```python
from build123d import *

# Parameters (mm, degrees)
F0_R     = 6.5
F1_DEPTH = 3


with BuildPart() as f1:
    # F0 (on Top) → F1 (new body)
    with BuildSketch(Plane.XY):
        with BuildLine():
            Line((0, 64.92969), (0, 105))
            ThreePointArc((0, 105), (-102.329905, 23.528505), (-45.860375, -94.455418))
            Line((-45.860375, -94.455418), (-26.848407, -75.44345))
            Line((-26.848407, -75.44345), (0, -75.44345))
            Line((0, -75.44345), (0, -45.946423))
            Line((0, -45.946423), (-4.373633, -45.946423))
            Line((-4.373633, -45.946423), (-8.012874, -43.948987))
            Line((-8.012874, -43.948987), (-8.012874, -40.483214))
            Line((-8.012874, -40.483214), (-7.424269, -39.663567))
            Line((-7.424269, -39.663567), (-23.331161, -42.38735))
            Line((-23.331161, -42.38735), (-33.173094, -41.479423))
            Line((-33.173094, -41.479423), (-35.896877, -38.101933))
            Line((-35.896877, -38.101933), (-34.589463, -35.37815))
            Line((-34.589463, -35.37815), (-37.494832, -32.944905))
            Line((-37.494832, -32.944905), (-40.373584, -28.384436))
            Line((-40.373584, -28.384436), (-39.757261, -25.662348))
            Line((-39.757261, -25.662348), (-30.409717, -16.543746))
            Line((-30.409717, -16.543746), (-28.680348, -16.543746))
            Line((-28.680348, -16.543746), (-27.497232, -17.393365))
            Line((-27.497232, -17.393365), (-27.497232, -5.479778))
            Line((-27.497232, -5.479778), (-32.618854, -5.479778))
            Line((-32.618854, -5.479778), (-32.618854, 5.955574))
            Line((-32.618854, 5.955574), (-27.497232, 5.955574))
            Line((-27.497232, 5.955574), (-27.497232, 30.408693))
            Line((-27.497232, 30.408693), (-30.054469, 38.053981))
            Line((-30.054469, 38.053981), (-16.39924, 35.148612))
            Line((-16.39924, 35.148612), (-21.810488, 39.03454))
            Line((-21.810488, 39.03454), (-21.810488, 43.537862))
            Line((-21.810488, 43.537862), (-24.057509, 47.911971))
            Line((-24.057509, 47.911971), (-25.507802, 47.911971))
            Line((-25.507802, 47.911971), (-27.497232, 52.08861))
            Line((-27.497232, 52.08861), (-26.29794, 52.65986))
            Line((-26.29794, 52.65986), (-27.144464, 54.437064))
            Line((-27.144464, 54.437064), (-23.446245, 56.198612))
            Line((-23.446245, 56.198612), (-21.478997, 54.78589))
            Line((-21.478997, 54.78589), (-20.486095, 54.78589))
            Line((-20.486095, 54.78589), (-20.000346, 54.437064))
            Line((-20.000346, 54.437064), (-14.9056, 55.777782))
            Line((-14.9056, 55.777782), (-14.033989, 61.988003))
            Line((-14.033989, 61.988003), (-10.583865, 57.266784))
            Line((-10.583865, 57.266784), (-4.373633, 58.90105))
            Line((-4.373633, 58.90105), (-4.373633, 60.244786))
            Line((-4.373633, 60.244786), (-2.230932, 60.244786))
            Line((-2.230932, 60.244786), (-2.230932, 64.92969))
            Line((-2.230932, 64.92969), (0, 64.92969))
        make_face()
        with Locations((-92.039506, -23.116552)):
            Circle(F0_R, mode=Mode.SUBTRACT)
        with Locations((-30.448022, 90.125876)):
            Circle(F0_R, mode=Mode.SUBTRACT)
        with BuildLine():
            ThreePointArc((45.134783, 94.804279), (23.136018, 102.419357), (0, 105))
            Line((0, 105), (0, 64.92969))
            Line((0, 64.92969), (3.688756, 64.92969))
            Line((3.688756, 64.92969), (3.688756, 60.499008))
            Line((3.688756, 60.499008), (5.722514, 60.499008))
            Line((5.722514, 60.499008), (5.722514, 58.683149))
            Line((5.722514, 58.683149), (11.814197, 56.869553))
            Line((11.814197, 56.869553), (15.854987, 62.496448))
            Line((15.854987, 62.496448), (16.254476, 55.777782))
            Line((16.254476, 55.777782), (22.025488, 54.02744))
            Line((22.025488, 54.02744), (22.527293, 54.726216))
            Line((22.527293, 54.726216), (23.500354, 54.02744))
            Line((23.500354, 54.02744), (24.861629, 55.923048))
            Line((24.861629, 55.923048), (28.822297, 54.02744))
            Line((28.822297, 54.02744), (27.664759, 52.415541))
            Line((27.664759, 52.415541), (28.711242, 52.000801))
            Line((28.711242, 52.000801), (27.023366, 47.741913))
            Line((27.023366, 47.741913), (25.696923, 48.04224))
            Line((25.696923, 48.04224), (23.37263, 43.575236))
            Line((23.37263, 43.575236), (23.37263, 39.03454))
            Line((23.37263, 39.03454), (21.266238, 38.49084))
            Line((21.266238, 38.49084), (21.266238, 37.256059))
            Line((21.266238, 37.256059), (18.796676, 35.512838))
            Line((18.796676, 35.512838), (31.907149, 37.800815))
            Line((31.907149, 37.800815), (31.300232, 30.408693))
            Line((31.300232, 30.408693), (31.300232, 5.955574))
            Line((31.300232, 5.955574), (36.421863, 5.955574))
            Line((36.421863, 5.955574), (36.419832, -5.479778))
            Line((36.419832, -5.479778), (31.300232, -5.33569))
            Line((31.300232, -5.33569), (31.300232, -15.820357))
            Line((31.300232, -15.820357), (31.300232, -16.543746))
            Line((31.300232, -16.543746), (32.996665, -16.543746))
            Line((32.996665, -16.543746), (42.221212, -27.097848))
            Line((42.221212, -27.097848), (42.221212, -27.860507))
            Line((42.221212, -27.860507), (35.611501, -35.45078))
            Line((35.611501, -35.45078), (36.628378, -39.227758))
            Line((36.628378, -39.227758), (30.418154, -41.987859))
            Line((30.418154, -41.987859), (26.169052, -41.987859))
            Line((26.169052, -41.987859), (12.985943, -39.954101))
            Line((12.985943, -39.954101), (9.281599, -39.954101))
            Line((9.281599, -39.954101), (9.281599, -43.948987))
            Line((9.281599, -43.948987), (5.795156, -45.946423))
            Line((5.795156, -45.946423), (0, -45.946423))
            Line((0, -45.946423), (0, -75.44345))
            Line((0, -75.44345), (25.397223, -75.44345))
            Line((25.397223, -75.44345), (44.40919, -94.455418))
            ThreePointArc((44.40919, -94.455418), (44.5367, -94.394607), (44.664128, -94.333625))
            ThreePointArc((44.664128, -94.333625), (88.130811, -55.593427), (104.274408, 0.348861))
            ThreePointArc((104.274408, 0.348861), (88.269743, 56.069866), (45.134783, 94.804279))
        make_face()
        with Locations((90.588322, -23.116552)):
            Circle(F0_R, mode=Mode.SUBTRACT)
        with Locations((28.571626, 90.125876)):
            Circle(F0_R, mode=Mode.SUBTRACT)
    extrude(amount=F1_DEPTH)


solid = f1.part
```
Could you check a few things on this model? Use its own coordinates, in mm. A direction names the side the tool comes from. Coordinates: 2 decimals unless noted, no trailing zeros. Order: outer loops, then holes, each group sorted by start corner. A loop starts at its lowest first (then second) coordinate and runs counter-clockwise, first axis right, second up. Notation, with made-up numbers: M 74.5,-17 L 91.5,-17 A19 cw 91.5,6 Z; hole C 50.5,16.5 d10. An arc over 180 degrees is marked long. Use one line per item in the form item = value. Start each with the question number.
1. For pin 1 (17 mm diameter, centred on x = 28.57, y = 90.13, fed in from -Z); pin 2 (0.9 mm diameter, centred on y = 14, z = 2, fed in from +X); pin 3 (0.9 mm diameter, centred on y = -12, z = 1, fed in from +X); pin 4 (1.5 mm diameter, centred on x = 11, z = 1.5, fed in from +Y), each with a flat end and sliding along its axis, tell me the tip position at first contact or that it passes through.
2. On a 3-axis mill with a long thin cutter (end or side, diameter ignored), from which of +Z, -Z, +X, -X, +Y, -Y can I reach the whole of each face in a straight line? I mean faces 3 (the flat face through (45, 7, 0)), 4 (the flat face through (-36.487, -85.083, 1.479)), 5 (the flat face through (37.544, -21.747, 1.479)). Say none if no direction works.
3. We'd pull the mould along X, two halves only. Please class faces 1 (the flat face through (45, 7, 3)), 2 (the flat face through (34.77, -84.816, 1.479)): +X half, -X half, draft (parallel to the pull), parting line (faces both ways), or undercut.
4. Suppose I cut it at C-C on z = 2.1. Count the separate pieces of the cut face and the enclosed holes in it, then the cut area to 3 significant figures.
5. Suppose I cut it at B-B on x = -63.5. Write out the boundary of the cut face in (y, z), then the cut area to 3 significant figures.
6. Suppose I cut it at A-A on y = 75. Write out the boundary of the cut face in (x, z).
7. Please list where these lines run through material, in increasing order: line 1 (X direction, y = 2.5, z = 0.6); line 2 (Y direction, x = -23, z = 2.85); line 3 (Y direction, x = 22, z = 2.15).
Geometry says:
q1.pin_1 = 0
q1.pin_2 = 103.44
q1.pin_3 = 103.6
q1.pin_4 = 104.5
q2.face_3 = -Z, +X, -X, +Y, -Y
q2.face_4 = +Z, -Z, -Y
q2.face_5 = +Z, -Z
q3.face_1 = draft
q3.face_2 = undercut
q4.separate_pieces = 1
q4.enclosed_holes = 5
q4.area = 25,700 mm^2
q5.outline = M -83.62,0 L 83.62,0 L 83.62,3 L -83.62,3 Z
q5.area = 502 mm^2
q6.outline = M -73.48,0 L 73.11,0 L 73.11,3 L -73.48,3 Z
q7.line_1 = -104.97 to -32.62, 36.42 to 104.25
q7.line_2 = -75.44 to -42.33, 36.55 to 45.85, 55.88 to 102.45
q7.line_3 = -75.44 to -41.34, 36.07 to 38.68, 54.04 to 102.67
